Geometry: final body of the model. Coordinates: model frame, mm. A direction names the side the tool comes from. Coordinates: 2 decimals unless noted, no trailing zeros. Order: outer loops, then holes, each group sorted by start corner. A loop starts at its lowest first (then second) coordinate and runs counter-clockwise, first axis right, second up. Notation, with made-up numbers: M -37.5,-29 L -14.5,-29 A31 cw -14.5,8 Z; hole C -17,-28.5 d2. An arc over 180 degrees is marked long. Use CSV: the item, a comma, the result in double quotes. Start each with the question number.
Q1. First-contact query: P1, Ø2, axis at y = 14.5, z = 6.5, coming from the -X side; P2, Ø0.8, axis at y = -24, z = -1, coming from the +X side; P3, Ø1.2, axis at y = -5, z = -1.5, coming from the -X side; P4, Ø25, axis at x = 9.5, y = -2.5, coming from the -Z side. Flat tips, straight axial feed; report the tip coordinate or a pass-through.
Q2. Section query C-C, the plane y = 33. Output: boundary loops of the cut face in (x, z), and give its area (3 significant figures).
Q3. Access query for faces 5 (the face through (38.5, 37, -1)), 6 (the face through (-19.185, -43.768, 15.379)), 7 (the face through (-70.5, -1, 17)), 8 (the face through (20, 9.43, -1.27)). Directions: +Z, -Z, +X, -X, +Y, -Y. A direction counts if a zero-diameter tool reaches every point of the face in a straight line with its end or side. Return the directions, or none.
Q4. Mould query, pull axis X, two halves, no side actions, for faces 1 (the face through (-2.825, 10.964, -1.268)), 2 (the face through (-1, -18, -2.5)), 3 (the face through (-73, -1, 17)), 4 (the face through (-28.5, 37, -1)). Classes: +X half, -X half, draft (parallel to the pull), parting line (faces both ways), or undercut.
Q5. Section query A-A, the plane x = 9.5. Output: boundary loops of the cut face in (y, z).
Q6. Section query B-B, the plane z = 3. Output: boundary loops of the cut face in (x, y), and give its area (3 significant figures).
Q7. Ray query, probe 1 along X at (y, z) = (-17, 16); probe 2 along Y at (x, z) = (-45, 24); probe 3 along Z at (x, y) = (56, 41). Return the intervals inside material, ascending.
Q8. Section query D-D, the plane z = 25.5. Output: boundary loops of the cut face in (x, y).
from build123d import *

# Parameters (mm, degrees)
SKETCH_W               = 141
SKETCH_H               = 85
PAD_DEPTH              = 28
THICKNESS_T            = 2.5
SKETCH001_R            = 1.5
POCKET_DEPTH           = 146.001
SKETCH003_W            = 51
SKETCH003_H            = 15
POCKET001_DEPTH        = 5
SKETCH004_W            = 67
SKETCH004_H            = 34.253407
POCKET002_DEPTH        = 15
SKETCH005_R            = 5
SKETCH005_W            = 22
SKETCH005_H            = 12
SKETCH005_W_2          = 14
POCKET003_DEPTH        = 5
SKETCH006_R            = 14
SKETCH006_R_2          = 1.5
POCKET004_DEPTH        = 5
POCKET005_DEPTH        = 5
LINEARPATTERN_COUNT    = 7
LINEARPATTERN_PITCH    = 7.5
POCKET006_DEPTH        = 5
LINEARPATTERN001_COUNT = 5
LINEARPATTERN001_PITCH = 7


with BuildPart() as part:
    # Sketch → Pad (new body)
    with BuildSketch(Plane.XY):
        Rectangle(SKETCH_W, SKETCH_H)
    extrude(amount=PAD_DEPTH)

    # Thickness
    thickness_openings = [part.faces().sort_by_distance(p)[0] for p in [
        (0, 0, 28),
    ]]
    offset(amount=THICKNESS_T, openings=thickness_openings)

    # Sketch001 → Pocket (cut, through all)
    with BuildSketch(Plane(origin=(-73, 0, 0), x_dir=(0, -1, 0), z_dir=(-1, 0, 0))):
        with Locations((-33, 22)):
            Circle(SKETCH001_R)
        with Locations((33, 22)):
            Circle(SKETCH001_R)
    extrude(amount=-POCKET_DEPTH, mode=Mode.SUBTRACT)

    # Sketch003 → Pocket001 (cut)
    with BuildSketch(Plane(origin=(-73, 0, 0), x_dir=(0, -1, 0), z_dir=(-1, 0, 0))):
        with Locations((-5, 7.5)):
            Rectangle(SKETCH003_W, SKETCH003_H)
    extrude(amount=-POCKET001_DEPTH, mode=Mode.SUBTRACT)

    # Sketch004 → Pocket002 (cut)
    with BuildSketch(Plane(origin=(0, 0, -2.5), x_dir=(1, 0, 0), z_dir=(0, 0, -1))):
        with Locations((5, -37.626703)):
            Rectangle(SKETCH004_W, SKETCH004_H)
    extrude(amount=-POCKET002_DEPTH, mode=Mode.SUBTRACT)

    # Sketch005 → Pocket003 (cut)
    with BuildSketch(Plane.XZ.offset(45)):
        with Locations((-15.5, 12)):
            Circle(SKETCH005_R)
        with Locations((5.5, 12)):
            Rectangle(SKETCH005_W, SKETCH005_H)
        with Locations((25.939165, 15)):
            Rectangle(SKETCH005_W_2, SKETCH005_H)
    extrude(amount=-POCKET003_DEPTH, mode=Mode.SUBTRACT)

    # Sketch006 → Pocket004 (cut)
    with BuildSketch(Plane(origin=(0, 0, -2.5), x_dir=(1, 0, 0), z_dir=(0, 0, -1))):
        with Locations((9.5, 2.5)):
            Circle(SKETCH006_R)
        with Locations((-2.5, 14.5)):
            Circle(SKETCH006_R_2)
        with Locations((21.5, 14.5)):
            Circle(SKETCH006_R_2)
        with Locations((21.5, -9.5)):
            Circle(SKETCH006_R_2)
        with Locations((-2.5, -9.5)):
            Circle(SKETCH006_R_2)
    extrude(amount=-POCKET004_DEPTH, mode=Mode.SUBTRACT)

    # Sketch007 → Pocket005 (cut)
    with BuildSketch(Plane(origin=(0, 0, -2.5), x_dir=(1, 0, 0), z_dir=(0, 0, -1))):
        with BuildLine():
            Line((-58.404976, 36.87695), (-58.404976, -13.12305))
            ThreePointArc((-62.404976, -13.12305), (-60.404976, -15.003782), (-58.404976, -13.12305))
            Line((-62.404976, -13.12305), (-62.404976, 36.87695))
            ThreePointArc((-58.404976, 36.87695), (-60.404976, 38.729629), (-62.404976, 36.87695))
        make_face()
    pocket005 = extrude(amount=-POCKET005_DEPTH, mode=Mode.SUBTRACT)

    # LinearPattern: Pocket005 ×7
    with Locations(*[(i * LINEARPATTERN_PITCH, 0, 0) for i in range(1, LINEARPATTERN_COUNT)]):
        add(pocket005, mode=Mode.SUBTRACT)

    # Sketch008 → Pocket006 (cut)
    with BuildSketch(Plane(origin=(0, 0, -2.5), x_dir=(1, 0, 0), z_dir=(0, 0, -1))):
        with BuildLine():
            Line((37.782045, 37), (37.782045, -13))
            ThreePointArc((33.782045, -13), (35.782045, -15), (37.782045, -13))
            Line((33.782045, -13), (33.782045, 37))
            ThreePointArc((37.782045, 37), (35.782045, 39), (33.782045, 37))
        make_face()
    pocket006 = extrude(amount=-POCKET006_DEPTH, mode=Mode.SUBTRACT)

    # LinearPattern001: Pocket006 ×5
    with Locations(*[(i * LINEARPATTERN001_PITCH, 0, 0) for i in range(1, LINEARPATTERN001_COUNT)]):
        add(pocket006, mode=Mode.SUBTRACT)


solid = part.part
Responses:
1,P1,"stops at x = 70.5"
1,P2,"stops at x = 72.93"
1,P3,"stops at x = -72.83"
1,P4,"passes through"
2,outline,"M -73,0 A2.5 ccw -70.5,-2.5 L -28.5,-2.5 L -28.5,0 L -70.5,0 L -70.5,20.5 L -73,20.5 Z; M -73,23.5 L -70.5,23.5 L -70.5,28 L -73,28 Z; M 38.5,-2.5 L 70.5,-2.5 A2.5 ccw 73,0 L 73,20.5 L 70.5,20.5 L 70.5,0 L 38.5,0 Z; M 70.5,23.5 L 73,23.5 L 73,28 L 70.5,28 Z"
2,area,"320 mm²"
3,face 5,"-Z, +Y"
3,face 6,"-Y"
3,face 7,"+Z"
3,face 8,"+Z, -Z"
4,face 1,"undercut"
4,face 2,"draft"
4,face 3,"-X half"
4,face 4,"undercut"
5,outline,"M -45,0 A2.5 ccw -42.5,-2.5 L -16.5,-2.5 L -16.5,0 L -42.5,0 L -42.5,6 L -45,6 Z; M -45,18 L -42.5,18 L -42.5,28 L -45,28 Z; M 11.5,-2.5 L 20.5,-2.5 L 20.5,0 L 11.5,0 Z; M 42.5,12.5 L 45,12.5 L 45,28 L 42.5,28 Z"
6,outline,"M -73,-42.5 A2.5 ccw -70.5,-45 L 70.5,-45 A2.5 ccw 73,-42.5 L 73,42.5 A2.5 ccw 70.5,45 L 38.5,45 L 38.5,42.5 L 70.5,42.5 L 70.5,-42.5 L -70.5,-42.5 L -70.5,-20.5 L -73,-20.5 Z; M -73,30.5 L -70.5,30.5 L -70.5,42.5 L -28.5,42.5 L -28.5,45 L -70.5,45 A2.5 ccw -73,42.5 Z"
6,area,"855 mm²"
7,probe 1,"x = -73 to -70.5, 70.5 to 73"
7,probe 2,"y = -45 to -42.5, 42.5 to 45"
7,probe 3,"z = -2.5 to 0"
8,outline,"M -73,-42.5 A2.5 ccw -70.5,-45 L 70.5,-45 A2.5 ccw 73,-42.5 L 73,42.5 A2.5 ccw 70.5,45 L -70.5,45 A2.5 ccw -73,42.5 Z; hole M -70.5,-42.5 L 70.5,-42.5 L 70.5,42.5 L -70.5,42.5 Z"
